Autodesk Inventor part; units mm, degrees
ref_plane "YZ Plane" through (0, 0, 0) normal (1, 0, 0) x (0, 1, 0)
ref_plane "XZ Plane" through (0, 0, 0) normal (0, 1, 0) x (-1, 0, 0)
ref_plane "XY Plane" through (0, 0, 0) normal (0, 0, 1) x (1, 0, 0)
sketch "Esquisse1" plane through (0, 0, 0) normal (0, 1, 0) x (-1, 0, 0)
  line L0 (55, 30) -> (-55, 30)
  line L1 (-55, 30) -> (-70, -30)
  line L2 (-70, -30) -> (70, -30)
  line L3 (70, -30) -> (55, 30)
  point P0 (0, 0)
  dimension "d0" = 140
  dimension "d1" = 110
  dimension "d2" = 60
  dimension "d3" = 70
  dimension "d4" = 55
  dimension "d5" = 30
extrude "Extrusion1" add sketch "Esquisse1" along normal blind 5
sketch "Esquisse2" plane through (0, 5, 0) normal (0, 1, 0) x (1, 0, 0)
  line L0 (-31.5, -27) -> (31.5, -27)
  line L1 (31.5, -27) -> (40, 30)
  line L2 (70, 30) -> (-70, 30)
  line L3 (-31.5, -27) -> (-40, 30)
  line L4 (40, 30) -> (-40, 30)
  line L5 (-55, -30) -> (55, -30)
  point P0 (0, 0)
  dimension "d8" = 80
  dimension "d9" = 63
  dimension "d10" = 31.5
  dimension "d11" = 40
  dimension "d12" = 3
extrude "Extrusion2" add sketch "Esquisse2" along normal blind 15
sketch "Esquisse3" plane through (-31.5, 5, 27) normal (0, 0, 1) x (1, 0, 0)
  circle A0 centre (31.5, 8) radius 4
  line L0 (0, 0) -> (0, 15)
  line L1 (63, 0) -> (63, 15)
  line L2 (71.5, 15) -> (-8.5, 15)
  point P0 (31.5, -5)
  dimension "d15" = 31.5
  dimension "d16" = 63
  dimension "d17" = 7
  dimension "d18" = 8
extrude "Extrusion3" cut sketch "Esquisse3" against normal blind 20
fillet "Congé1" radius 5 4 edges at (31.5, 12.5, 27) (-31.5, 12.5, 27) (55, 2.5, 30) (-55, 2.5, 30)
sketch "Esquisse5" plane through (0, 20, 0) normal (0, 1, 0) x (1, 0, 0)
  circle A0 centre (-59.5, 18.5) radius 1.25
  circle A1 centre (59.5, 18.5) radius 1.25
  circle A2 centre (20.5, -16) radius 1.25
  circle A3 centre (-20.5, -16) radius 1.25
  line L0 (-40, 30) -> (-70, 30)
  line L1 (70, 30) -> (40, 30)
  point P0 (0, 0)
  dimension "d22" = 2.5
  dimension "d23" = 2.5
  dimension "d24" = 2.5
  dimension "d25" = 2.5
  dimension "d26" = 119
  dimension "d27" = 41
  dimension "d28" = 59.5
  dimension "d30" = 20.5
  dimension "d31" = 34.5
  dimension "d32" = 11.5
  dimension "d33" = 11.5
  dimension "d34" = 34.5
extrude "Extrusion4" cut sketch "Esquisse5" against normal through all
equation "\"d15\" = 0.5 * d16"
equation "\"d23\" = d22"
equation "\"d24\" = d22"
equation "\"d25\" = d22"
equation "\"d33\" = d32"
equation "\"d34\" = d31"
properties part number "Pont_arriere" material "Bois (Cerisier)"
The listing builds one solid part. Answer for the finished solid, in the listing's coordinates (mm). A direction names the side the tool comes from. Round coordinates to 2 decimals unless told otherwise and drop trailing zeros. Loops run counter-clockwise (first coordinate to the right, second up) from the corner with the lowest first, then second, coordinate; pieces in that order, holes last. Notation, with made-up numbers: M -1.5,3.5 L 40.5,3.5 A32 cw 40.5,38.5 Z; hole C 39,-5.5 d3. An arc over 180 degrees is marked long. Return JSON: item names as keys, results as strings.
Q1. Find section B-B, the plane y = 2. Determine the outline of the cut face in (x, z), plus the area to 3 significant figures.
Results list:
{"outline": "M -70,-30 L 70,-30 L 55.95,26.21 A5 ccw 51.1,30 L -51.1,30 A5 ccw -55.95,26.21 Z; hole C -59.5,-18.5 d2.5; hole C -20.5,16 d2.5; hole C 20.5,16 d2.5; hole C 59.5,-18.5 d2.5", "area": "7,470 mm2"}
Q2. The mould has two halves that part along Y. Classify faces 5 (the face through (-0.521, 16.966, 17.14)), 6 (the face through (-30.492, 12.605, 25.755)), 7 (the face through (1, 0, 0)): released by +Y, released by -Y, zero draft, split by the parting line, or undercut.
Results list:
{"face 5": "undercut", "face 6": "zero draft", "face 7": "released by -Y"}
Q3. Which of the six approach directions +Z, -Z, +X, -X, +Y, -Y give full straight-line access (tool end or side, diameter ignored) to faces 1 (the face through (-36.013, 12.395, -3.262)), 2 (the face through (0, 7, 27)), 3 (the face through (0, 13, 7)), 4 (the face through (30.417, 12.605, 25.82))?
Results list:
{"face 1": "+Z, -X, +Y", "face 2": "+Z, +X, -X, +Y", "face 3": "+Z", "face 4": "+Z, +X, +Y"}
Q4. Each of these flat-tipped pins is pushed along its axis until it touches: pin 1 Ø5 at (x, y) = (-49.5, 9.5) entering from -Z (3 decimals); pin 2 Ø8 at (x, y) = (9.5, 7) entering from +Z; pin 3 Ø3 at (y, z) = (13.5, -16) entering from +X; pin 4 Ø2.5 at (x, y) = (2, 15) entering from +Z. Where does it stop, or does it pass through?
Results list:
{"pin 1": "passes through", "pin 2": "stops at z = 30", "pin 3": "stops at x = 38.14", "pin 4": "stops at z = 27"}
Q5. Find section C-C, the plane z = 16. Determine the outline of the cut face in (x, y).
Results list:
{"outline": "M -58.5,0 L -21.75,0 L -21.75,20 L -33.14,20 L -33.14,5 L -58.5,5 Z; M -19.25,0 L 19.25,0 L 19.25,20 L -19.25,20 Z; M 21.75,0 L 58.5,0 L 58.5,5 L 33.14,5 L 33.14,20 L 21.75,20 Z; hole C 0,13 d8"}
Q6. Find section D-D, the plane y = 13. Determine the outline of the cut face in (x, z).
Results list:
{"outline": "M -40,-30 L 40,-30 L 32.14,22.74 A5 ccw 27.19,27 L 4,27 L 4,7 L -4,7 L -4,27 L -27.19,27 A5 ccw -32.14,22.74 Z; hole C -20.5,16 d2.5; hole C 20.5,16 d2.5"}
Q7. Find section A-A, the plane x = -59.5. Determine the outline of the cut face in (y, z), plus the area to 4 significant figures.
Results list:
{"outline": "M 0,-30 L 5,-30 L 5,-19.75 L 0,-19.75 Z; M 0,-17.25 L 5,-17.25 L 5,12 L 0,12 Z", "area": "197.5 mm2"}
Q8. Find the intervals of material crossed by line 1 along Z through (x, y) = (20.5, 7.25); line 2 along Y through (x, z) = (0, 13.5); line 3 along X through (y, z) = (1.3, -18.5) (3 decimals), in increasing order. Write a range as from..to.
Results list:
{"line 1": "z = -30..14.75, 17.25..27", "line 2": "y = 0..9, 17..20", "line 3": "x = -67.125..-60.75, -58.25..58.25, 60.75..67.125"}
